For this review, take the finished solid that the model builds, in its own axes (mm). A direction names the side the tool comes from. Coordinates: 2 decimals unless noted, no trailing zeros. Write each loop counter-clockwise with the first axis right and the second up, starting at its lowest first coordinate (ties: lowest second). Pieces come first, ordered by that corner, then holes.
1) Mouldability with a two-part tool opening along Z and no side actions: class faces 5 (the face through (61, 4, 14.667)), 6 (the face through (20, 66, 179.667)), 7 (the face through (0, 61, 167)), 8 (the face through (61, 4, 30.167)) as pulls with the +Z half, pulls with the -Z half, needs draft (parallel to the pull), parting line crosses it, or undercut.
2) To check wall thickness, follow line 1 along Y through (x, z) = (54, 138); line 2 along Z through (x, y) = (56, 1); line 3 along Z through (x, y) = (17.5, 177.5). State the ranges of each line that lie inside material, in increasing order.
3) We need section A-A on z = 89. Write out the cut boundary in (x, y).
4) We need section B-B on x = 78. Give the number of separate pieces and of enclosed holes in the cut face, then the cut area to 3 significant figures.
5) We need section D-D on z = 24.5. Write out the cut boundary in (x, y).
6) Insertion check: P1, Ø4, axis at y = 120.5, z = 172.5, coming from the +X side; P2, Ø2.5, axis at x = 25, z = 170, coming from the -Y side; P3, Ø2, axis at x = 12.5, y = 42, coming from the -Z side. Each pin has a flat end and moves straight along its axis. Give the tip position at first contact, or say it passes through.
7) For faces 1 (the face through (18, 31, 171)), 2 (the face through (51.66, 32.16, 163.09)), 3 (the face through (64.45, 90.96, 170.72)), 4 (the face through (59, 19.333, -52)), list the 3-axis set-ups (+Z, -Z, +X, -X, +Y, -Y) from which the entire face can be reached by the end or side of a thin tool; tool diameter is ignored.
from build123d import *

# Parameters (mm, degrees)
EXTRUDE_1_DEPTH     = 120
SKETCH_2_W          = 15.5
SKETCH_2_H          = 10
CUT_EXTRUDE_1_DEPTH = 324.916484435
CUT_EXTRUDE_2_DEPTH = 40
CUT_EXTRUDE_3_DEPTH = 40
FILLET_16_R         = 5
EXTRUDE_2_DEPTH     = 239
EXTRUDE_3_DEPTH     = 18
FILLET_17_R         = 5


with BuildPart() as part:
    # 草圖1 → 填料-伸長1 (new body)
    with BuildSketch(Plane(origin=(0, 0, 0), x_dir=(0, 0, -1), z_dir=(1, 0, 0))):
        Polygon((-179.666666667, 241.333333333), (-179.666666667, -8.666666667), (59.333333333, -8.666666667), (59.333333333, 9.333333333), (59.333333333, 19.333333333), (44.333333333, 19.333333333), (44.333333333, 9.333333333), (-161.666666667, 9.333333333), (-161.666666667, 241.333333333), align=None)
    extrude(amount=EXTRUDE_1_DEPTH)

    # 草圖2 → 除料-伸長1 (cut, through all)
    with BuildSketch(Plane(origin=(120, 0, 0), x_dir=(0, 0, -1), z_dir=(1, 0, 0))):
        with Locations((-22.416666667, 4.333333333)):
            Rectangle(SKETCH_2_W, SKETCH_2_H)
    extrude(amount=-CUT_EXTRUDE_1_DEPTH, mode=Mode.SUBTRACT)

    # 草圖4 → 除料-伸長2 (cut)
    with BuildSketch(Plane.XY.offset(179.666666667)):
        Polygon((120, 241.333333333), (18, 241.333333333), (120, 9.333333333), align=None)
    extrude(amount=-CUT_EXTRUDE_2_DEPTH, mode=Mode.SUBTRACT)

    # 草圖5 → 除料-伸長3 (cut)
    with BuildSketch(Plane.XY.offset(179.666666667)):
        Polygon((36, 155.668785671), (100.337138528, 9.333333333), (18, 9.333333333), (18, 155.668785671), align=None)
    extrude(amount=-CUT_EXTRUDE_3_DEPTH, mode=Mode.SUBTRACT)

    # 圓角16
    # the kernel refuses this fillet: 5 mm, written as the material it takes off along each edge
    with BuildSketch(Plane(origin=(14.736369898, 236.333333333, 166.666666667), x_dir=(0.9154313590233789, 0.40247413198441667, 0), z_dir=(0, 0, -1))) as fillet_16_piece_1_section:
        Polygon((0, 0), (FILLET_16_R, 0), (FILLET_16_R, -FILLET_16_R * 0.652726020499), (FILLET_16_R * 0.402474131984, -FILLET_16_R * 0.915431359023), align=None)
    fillet_16_piece_1 = extrude(amount=FILLET_16_R, mode=Mode.PRIVATE)
    fillet_16_piece_1 = fillet_16_piece_1 - Plane(origin=(14.736369898, 236.333333333, 166.666666667), x_dir=(-0.5465921093537591, -0.8373989885306815, 0), z_dir=(0, 0, -1)) * Sphere(FILLET_16_R, mode=Mode.PRIVATE)
    add(fillet_16_piece_1, mode=Mode.SUBTRACT)
    with BuildSketch(Plane(origin=(14.736369898, 236.333333333, 174.666666667), x_dir=(0, 1, 0), z_dir=(0, 0, 1))) as fillet_16_piece_2_section:
        Polygon((0, 0), (FILLET_16_R, 0), (FILLET_16_R, -FILLET_16_R * 0.652726020499), (FILLET_16_R * 0.402474131984, -FILLET_16_R * 0.915431359023), align=None)
    fillet_16_piece_2 = extrude(amount=FILLET_16_R, mode=Mode.PRIVATE)
    fillet_16_piece_2 = fillet_16_piece_2 - Plane(origin=(14.736369898, 236.333333333, 174.666666667), x_dir=(-0.5465921093537591, -0.8373989885306815, 0), z_dir=(0, 0, 1)) * Sphere(FILLET_16_R, mode=Mode.PRIVATE)
    add(fillet_16_piece_2, mode=Mode.SUBTRACT)
    with BuildSketch(Plane(origin=(-12.5, 241.333333333, 161.666666667), x_dir=(0, 0, 1), z_dir=(1, 0, 0)), Plane(origin=(-12.5, 241.333333333, 179.666666667), x_dir=(0, -1, 0), z_dir=(1, 0, 0))) as fillet_16_piece_3:
        with BuildLine():
            CenterArc((FILLET_16_R, FILLET_16_R), FILLET_16_R, 180, 90)
            Line((0, FILLET_16_R), (0, 0))
            Line((0, 0), (FILLET_16_R, 0))
        make_face()
    extrude(amount=27.236369898, mode=Mode.SUBTRACT)
    with BuildSketch(Plane(origin=(18, 241.333333333, 174.666666667), x_dir=(-1, 0, 0), z_dir=(0, 0, -1))) as fillet_16_piece_4:
        with BuildLine():
            CenterArc((FILLET_16_R * 0.652726020499, -FILLET_16_R), FILLET_16_R, 90, 66.267060196)
            Line((-FILLET_16_R * 0.262705338524, -FILLET_16_R * 0.597525868016), (0, 0))
            Line((0, 0), (FILLET_16_R * 0.652726020499, 0))
        make_face()
    extrude(amount=8, mode=Mode.SUBTRACT)
    with BuildSketch(Plane(origin=(19.313526693, 238.345703993, 161.666666667), x_dir=(0, 0, 1), z_dir=(0.40247413198441667, -0.9154313590233789, 0))) as fillet_16_piece_5_section:
        with BuildLine():
            CenterArc((FILLET_16_R, FILLET_16_R), FILLET_16_R, 180, 90)
            Line((0, FILLET_16_R), (0, 0))
            Line((0, 0), (FILLET_16_R, 0))
        make_face()
    fillet_16_piece_5 = extrude(amount=262.668806653, mode=Mode.PRIVATE)
    fillet_16_piece_5 = split(fillet_16_piece_5, bisect_by=Plane(origin=(68.522420019, 9.333333333, 162.799850977), z_dir=(0, 1, 0)), keep=Keep.TOP, mode=Mode.PRIVATE)
    add(fillet_16_piece_5, mode=Mode.SUBTRACT)
    with BuildSketch(Plane(origin=(19.313526693, 238.345703993, 179.666666667), x_dir=(-0.9154313590233789, -0.40247413198441667, 5.6843418860808026e-15), z_dir=(0.40247413198441667, -0.9154313590233789, 0))) as fillet_16_piece_6:
        with BuildLine():
            CenterArc((FILLET_16_R, FILLET_16_R), FILLET_16_R, 180, 90)
            Line((0, FILLET_16_R), (0, 0))
            Line((0, 0), (FILLET_16_R, 0))
        make_face()
    extrude(amount=262.668806653, mode=Mode.SUBTRACT)

    # 草圖8 → 填料-伸長2 (add)
    with BuildSketch(Plane.XY.offset(179.666666667)):
        with BuildLine():
            ThreePointArc((110.17, -13.666666712), (115.684274668, -12.344840676), (120, -8.666666667))
            Line((120, -8.666666667), (110.17, -8.666666667))
            Line((110.17, -8.666666667), (110.17, -13.666666667))
        make_face()
        with BuildLine():
            Line((110.17, -13.666666667), (110.17, -8.666666667))
            Line((110.17, -8.666666667), (100.34, -8.666666667))
            ThreePointArc((100.34, -8.666666667), (104.655725332, -12.344840676), (110.17, -13.666666712))
        make_face()
        with BuildLine():
            ThreePointArc((110.17, -13.666666712), (115.684274668, -12.344840676), (120, -8.666666667))
            Line((120, -8.666666667), (110.17, -8.666666667))
            Line((110.17, -8.666666667), (110.17, -13.666666667))
        make_face()
        with BuildLine():
            Line((110.17, -13.666666667), (110.17, -8.666666667))
            Line((110.17, -8.666666667), (100.34, -8.666666667))
            ThreePointArc((100.34, -8.666666667), (104.655725332, -12.344840676), (110.17, -13.666666712))
        make_face()
    extrude(amount=-EXTRUDE_2_DEPTH)

    # 草圖9 → 填料-伸長3 (add)
    with BuildSketch(Plane.XY.offset(179.666666667)):
        Polygon((18, 63.079938443), (100.337138528, 9.333333333), (93.709875708, 24.407107589), (22.919522331, 70.616403134), (18, 73.827683351), align=None)
        Polygon((18, 52.332193536), (83.872125352, 9.333333333), (100.337138528, 9.333333333), (18, 63.079938443), align=None)
        Polygon((100.337138528, 9.333333333), (83.872125352, 9.333333333), (95.417616197, 1.796868643), align=None)
        Polygon((93.711170014, 24.406262715), (100.337138528, 9.333333333), (105.256660859, 16.869798024), align=None)
        Polygon((10.463535309, 67.999460774), (18, 63.079938443), (18, 73.827683351), (15.38305764, 75.535925465), align=None)
        Polygon((13.080477669, 55.543473753), (18, 52.332193536), (18, 63.079938443), align=None)
    extrude(amount=-EXTRUDE_3_DEPTH)

    # 圓角17
    fillet_17_edges = [part.edges().sort_by_distance(p)[0] for p in [
        (18, 30.832763435, 179.666666667),
        (18, 30.832763435, 161.666666667),
        (64.854937854, 90.03794663, 179.666666667),
        (64.854937854, 90.03794663, 161.666666667),
        (50.936062676, 30.832763435, 179.666666667),
        (55.854937854, 49.11739547, 179.666666667),
        (55.854937854, 49.11739547, 161.666666667),
        (50.936062676, 30.832763435, 161.666666667),
        (18, 114.748234511, 161.666666667),
        (27, 155.668785671, 161.666666667),
        (27, 155.668785671, 179.666666667),
        (18, 114.748234511, 179.666666667),
        (50.936062676, 9.333333333, 179.666666667),
    ]]
    fillet(fillet_17_edges, radius=FILLET_17_R)


solid = part.part
Result:
1. face 5: undercut
1. face 6: pulls with the +Z half
1. face 7: needs draft
1. face 8: undercut
2. line 1: y = -8.67 to 9.33
2. line 2: z = -59.33 to 14.67, 30.17 to 179.67
2. line 3: z = 161.67 to 179.67
3. outline: (0, -8.67) - (100.34, -8.67) arc R12.16 ccw to (120, -8.67) - (120, 9.33) - (0, 9.33) - close
4. separate pieces: 3
4. enclosed holes: 0
4. area: 5,400 mm2
5. outline: (0, -8.67) - (100.34, -8.67) arc R12.16 ccw to (120, -8.67) - (120, -0.67) - (0, -0.67) - close
6. P1: stops at x = 72
6. P2: stops at y = -8.67
6. P3: stops at z = 161.67
7. face 1: +Z
7. face 2: none
7. face 3: +Z, -Z
7. face 4: -Z, +X, -X, +Y
